```python
from build123d import *

# Parameters (mm, degrees)
SKETCH2_R   = 45.59
SKETCH2_R_2 = 44.09


with BuildPart() as part:
    # Sweep1: sweep along a path in Sketch1
    with BuildLine(Plane(origin=(0, 0, 0), x_dir=(1, 0, 0), z_dir=(0, 1, 0))) as sweep1_path:
        Line((0, 0), (0, 140))
        ThreePointArc((0, 140), (-46.86291501, 253.13708499), (-160, 300))
        Line((-160, 300), (-1840, 300))
        ThreePointArc((-1840, 300), (-1953.13708499, 346.86291501), (-2000, 460))
        Line((-2000, 460), (-2000, 700))
    # Sketch2 → Sweep1 (sweep)
    with BuildSketch(Plane.XY):
        Circle(SKETCH2_R)
        Circle(SKETCH2_R_2, mode=Mode.SUBTRACT)
    sweep(path=sweep1_path.line)


solid = part.part
```
For this review, take the finished solid that the model builds, in its own axes (mm). A direction names the side the tool comes from. Coordinates: 2 decimals unless noted, no trailing zeros. Write each loop counter-clockwise with the first axis right and the second up, starting at its lowest first coordinate (ties: lowest second). Pieces come first, ordered by that corner, then holes. Notation, with made-up numbers: (75, 80) - (82, 80) arc R28 ccw to (82, 101) - close; hole circle Ø8 at (5.25, -12). An arc over 180 degrees is marked (long way). Answer in a Markdown table with one row per item. Add a question column.
Q1. We need section B-B, the plane x = -1060. State the section outline as (y, z) points, and give its area (3 significant figures).
Q2. Tool access review of faces 1 (the flat face through (-23.9, 37.4, 0)), 2 (the cylindrical face through (-44.047, -1.939, -70.98)): name each direction out of +Z, -Z, +X, -X, +Y, -Y from which nothing blocks a thin tool from reaching the whole face with its end or side.
Q3. For probe 1 along Z at (x, y) = (-613.5, -6); probe 2 along X at (y, z) = (0, -546); probe 3 along X at (y, z) = (-5, -634), list the stretches that pass through material, from the lowest coordinate up.
Q4. We need section C-C, the plane z = -525. State the section outline as (x, y) points, and give its area (3 significant figures).
Q5. For P1, Ø12, axis at y = -36.5, z = -101, coming from the +X side; P2, Ø5, axis at y = -25, z = -132.5, coming from the +X side; P3, Ø3, axis at x = -1285, y = -21, coming from the -Z side, all flat-tipped, find the tip position at first contact; note any pin that passes through.
Q6. We need section A-A, the plane y = 0. State the section outline as (x, z) points.
Q7. Draft analysis for pull direction X (two halves, no side actions). For faces 3 (the cylindrical face through (-1011.76, 26.828, -265.012)), 4 (the cylindrical face through (-1957.946, -13.243, -581.68)), 5 (the cylindrical face through (-1011.76, -2.005, -254.454)), 6 (the cylindrical face through (-1957.886, 17.461, -581.68)), state which applies: +X half, -X half, draft (parallel to the pull), parting line (faces both ways), or undercut.
Answer list:
| question | item | result |
|---|---|---|
| 1 | outline | circle Ø91.18 at (0, -300); hole circle Ø88.18 at (0, -300) |
| 1 | area | 423 mm2 |
| 2 | face 1 | +Z, +X, -X, +Y, -Y |
| 2 | face 2 | +Z |
| 3 | probe 1 | z = -345.19 to -343.68, -256.32 to -254.81 |
| 3 | probe 2 | x = -2045.59 to -2044.09, -1955.91 to -1954.41 |
| 3 | probe 3 | x = -2045.31 to -2043.81, -1956.19 to -1954.69 |
| 4 | outline | circle Ø91.18 at (-2000, 0); hole circle Ø88.18 at (-2000, 0) |
| 4 | area | 423 mm2 |
| 5 | P1 | stops at x = 33.89 |
| 5 | P2 | stops at x = 39.65 |
| 5 | P3 | stops at z = -341.21 |
| 6 | outline | (-2045.59, -700) - (-2044.09, -700) - (-2044.09, -460) arc R204.09 cw to (-1840, -255.91) - (-160, -255.91) arc R115.91 ccw to (-44.09, -140) - (-44.09, 0) - (-45.59, 0) - (-45.59, -140) arc R114.41 cw to (-160, -254.41) - (-1840, -254.41) arc R205.59 ccw to (-2045.59, -460) - close; (-1955.91, -700) - (-1954.41, -700) - (-1954.41, -460) arc R114.41 cw to (-1840, -345.59) - (-160, -345.59) arc R205.59 ccw to (45.59, -140) - (45.59, 0) - (44.09, 0) - (44.09, -140) arc R204.09 cw to (-160, -344.09) - (-1840, -344.09) arc R115.91 ccw to (-1955.91, -460) - close |
| 7 | face 3 | undercut |
| 7 | face 4 | undercut |
| 7 | face 5 | draft |
| 7 | face 6 | parting line |
